from build123d import *

# Parameters (mm, degrees)
F0_W      = 152.4
F0_H      = 76.2
F1_DEPTH  = 5.08
F2_T      = -2.54
F3_W      = 12.7
F3_H      = 12.7
F4_DEPTH  = 3.81
F4_TAPER  = 15
F5_W      = 12.7
F5_H      = 12.7
F6_DEPTH  = 3.81
F6_TAPER  = 15
F7_W      = 12.7
F7_H      = 12.7
F8_DEPTH  = 3.81
F8_TAPER  = 15
F9_W      = 12.7
F9_H      = 12.7
F10_DEPTH = 3.81
F10_TAPER = 15
F11_W     = 12.7
F11_H     = 12.7
F13_DEPTH = 3.81
F13_TAPER = 15


with BuildPart() as f1:
    # F0 (on Top) → F1 (new body)
    with BuildSketch(Plane.XY):
        with Locations((-40.1846427969, -17.2922080383)):
            Rectangle(F0_W, F0_H)
    extrude(amount=F1_DEPTH)

    # F2
    f2_openings = [f1.faces().sort_by_distance(p)[0] for p in [
        (-40.184643, -17.292208, 5.08),
    ]]
    offset(amount=F2_T, openings=f2_openings)

    # F3 (on face) → F4 (join)
    with BuildSketch(Plane.XY.offset(2.54)):
        with Locations((-107.4946427969, 11.9177919617)):
            Rectangle(F3_W, F3_H)
    extrude(amount=F4_DEPTH, taper=F4_TAPER)

    # F5 (on face) → F6 (join)
    with BuildSketch(Plane.XY.offset(2.54)):
        with Locations((-107.4946427969, -0.7822080383)):
            Rectangle(F5_W, F5_H)
    extrude(amount=F6_DEPTH, taper=F6_TAPER)

    # F7 (on face) → F8 (join)
    with BuildSketch(Plane.XY.offset(2.54)):
        with Locations((-107.4946427969, -13.4822080383)):
            Rectangle(F7_W, F7_H)
    extrude(amount=F8_DEPTH, taper=F8_TAPER)

    # F9 (on face) → F10 (join)
    with BuildSketch(Plane.XY.offset(2.54)):
        with Locations((-107.4946427969, -26.1822080383)):
            Rectangle(F9_W, F9_H)
    extrude(amount=F10_DEPTH, taper=F10_TAPER)

    # F11 (on face) → F13 (join)
    with BuildSketch(Plane.XY.offset(2.54)):
        with Locations((-107.4946427969, -38.8822080383)):
            Rectangle(F11_W, F11_H)
    extrude(amount=F13_DEPTH, taper=F13_TAPER)


solid = f1.part
Read the model definition and answer for the solid it produces. Units are mm, in the model's axes. A direction names the side the tool comes from. Round coordinates to 2 decimals unless told otherwise and drop trailing zeros. Order: outer loops, then holes, each group sorted by start corner. A loop starts at its lowest first (then second) coordinate and runs counter-clockwise, first axis right, second up. Notation, with made-up numbers: (63, 11.25) - (83, 11.25) arc R24 ccw to (83, 35.25) - close; hole circle Ø5 at (37.5, -25.5). An arc over 180 degrees is marked (long way). Use one line per item in the form item = value. Start each with the question number.
(1) For faces 1 (the face through (-108, -13, 6.35)), 2 (the face through (-101.65, -0.69, 4.42)), determine the directions among +Z, -Z, +X, -X, +Y, -Y from which every point of the face is accessible in a straight line to the end or side of a thin tool.
(2) Find the intervals of material crossed by line 1 along X through (y, z) = (-16.5, 4.75); line 2 along Y through (x, z) = (-37, 4); line 3 along X through (y, z) = (-37, 4), in increasing order. Write a range as from..to.
(3) Determine the mould class of faces 3 (the face through (-101.65, -13.39, 4.42)), 4 (the face through (36.015, -18, 3)), 5 (the face through (-41, -55.392, 3)), 6 (the face through (-113.34, -0.87, 4.42)) for opening direction X: +X half, -X half, draft (parallel to the pull), parting line (faces both ways), or undercut.
(4) The part is cut by section C-C (y = -0.5). Give the vertices of the cut face in (x, z).
(5) Flat-ended cylindrical pins translate along their axes: pin 1 Ø2 at (y, z) = (-35, 5.5) entering from +X; pin 2 Ø23 at (x, y) = (-42.5, -9) entering from +Z. Find the tip coordinate at first contact, or state that the pin passes through.
(6) The part is cut by section A-A (z = 4). Give the vertices of the cut face in (x, y), then the cut area to 3 significant figures.
(7) The part is cut by section B-B (x = 3.5). Give the vertices of the cut face in (y, z), then the cut area to 3 significant figures.
Checked values:
q1.face_1 = +Z, +X, -X, +Y, -Y
q1.face_2 = +Z
q2.line_1 = -116.38..-113.84, -113.25..-101.74, 33.48..36.02
q2.line_2 = -55.39..-52.85, 18.27..20.81
q2.line_3 = -116.38..-113.84, -113.45..-101.54, 33.48..36.02
q3.face_3 = undercut
q3.face_4 = +X half
q3.face_5 = draft
q3.face_6 = undercut
q4.outline = (-116.38, 0) - (36.02, 0) - (36.02, 5.08) - (33.48, 5.08) - (33.48, 2.54) - (-101.14, 2.54) - (-102.17, 6.35) - (-112.82, 6.35) - (-113.84, 2.54) - (-113.84, 5.08) - (-116.38, 5.08) - close
q5.pin_1 = 36.02
q5.pin_2 = 2.54
q6.outline = (-116.38, -55.39) - (36.02, -55.39) - (36.02, 20.81) - (-116.38, 20.81) - close; (-113.45, -44.84) - (-101.54, -44.84) - (-101.54, -32.92) - (-113.45, -32.92) - close; (-113.45, -32.14) - (-101.54, -32.14) - (-101.54, -20.22) - (-113.45, -20.22) - close; (-113.45, -19.44) - (-101.54, -19.44) - (-101.54, -7.52) - (-113.45, -7.52) - close; (-113.45, -6.74) - (-101.54, -6.74) - (-101.54, 5.18) - (-113.45, 5.18) - close; (-113.45, 5.96) - (-101.54, 5.96) - (-101.54, 17.88) - (-113.45, 17.88) - close; hole (-113.84, -52.85) - (33.48, -52.85) - (33.48, 18.27) - (-113.84, 18.27) - close
q6.area = 1,850 mm^2
q7.outline = (-55.39, 0) - (20.81, 0) - (20.81, 5.08) - (18.27, 5.08) - (18.27, 2.54) - (-52.85, 2.54) - (-52.85, 5.08) - (-55.39, 5.08) - close
q7.area = 206 mm^2
